CAD build for the part. Positions are in the model's coordinates, mm. A direction names the side the tool comes from. Round coordinates to 2 decimals unless told otherwise and drop trailing zeros. Loops run counter-clockwise (first coordinate to the right, second up) from the corner with the lowest first, then second, coordinate; pieces in that order, holes last.
from build123d import *

# Parameters (mm, degrees)
CROQUIS1_R              = 4.5
SALIENTE_EXTRUIR1_DEPTH = 12.5
SALIENTE_EXTRUIR2_START = 5
SALIENTE_EXTRUIR2_DEPTH = 5
CROQUIS4_R              = 2.5
SALIENTE_EXTRUIR3_DEPTH = 20
CORTAR_EXTRUIR1_DEPTH   = 3
SALIENTE_EXTRUIR4_START = -5
SALIENTE_EXTRUIR4_DEPTH = 5
CROQUIS7_W              = 256.925453937
CROQUIS7_H              = 4
CORTAR_EXTRUIR2_DEPTH   = 10
SALIENTE_EXTRUIR6_DEPTH = 5
CROQUIS9_W              = 256.997943919
CROQUIS9_H              = 4
CORTAR_EXTRUIR3_DEPTH   = 10
CROQUIS10_R             = 2.5
SALIENTE_EXTRUIR7_DEPTH = 25
SALIENTE_EXTRUIR9_DEPTH = 50
MATRIZL1_COUNT          = 2
MATRIZL1_PITCH          = 100
MATRIZL1_COPY_1_DEPTH   = 50


with BuildPart() as part:
    # Croquis1 → Saliente-Extruir1 (new, symmetric)
    with BuildSketch(Plane.XY):
        Circle(CROQUIS1_R)
    extrude(amount=SALIENTE_EXTRUIR1_DEPTH, both=True)

    # Croquis2 → Saliente-Extruir2 (add)
    with BuildSketch(Plane.XY.offset(12.5).offset(SALIENTE_EXTRUIR2_START)):
        with BuildLine():
            Line((0, 4.5), (120, 4.5))
            ThreePointArc((120, 4.5), (124.5, 0), (120, -4.5))
            Line((120, -4.5), (0, -4.5))
            ThreePointArc((0, -4.5), (-4.5, 0), (0, 4.5))
        make_face()
    saliente_extruir2 = extrude(amount=-SALIENTE_EXTRUIR2_DEPTH)

    # Simetría1: Saliente-Extruir2 across plane
    add(saliente_extruir2.mirror(Plane.XY))

    # Croquis4 → Saliente-Extruir3 (add, symmetric)
    with BuildSketch(Plane.XY):
        with Locations(Location((120, 0, 0), (0, 0, 180))):
            Circle(CROQUIS4_R)
    extrude(amount=SALIENTE_EXTRUIR3_DEPTH, both=True)

    # Croquis5 → Cortar-Extruir1 (cut)
    with BuildSketch(Plane.XY.offset(17.5)):
        with BuildLine():
            Line((0, 2), (90, 2))
            ThreePointArc((90, 2), (92, 0), (90, -2))
            Line((90, -2), (0, -2))
            ThreePointArc((0, -2), (-2, 0), (0, 2))
        make_face()
    cortar_extruir1 = extrude(amount=-CORTAR_EXTRUIR1_DEPTH, mode=Mode.SUBTRACT)

    # Simetría2: Cortar-Extruir1 across plane
    add(cortar_extruir1.mirror(Plane.XY), mode=Mode.SUBTRACT)

    # Croquis6 → Saliente-Extruir4 (add)
    with BuildSketch(Plane(origin=(0, 0, -17.5), x_dir=(-1, 0, 0), z_dir=(0, 0, -1)).offset(SALIENTE_EXTRUIR4_START)):
        with BuildLine():
            Line((0, 4.5), (210, 4.5))
            Line((210, 4.5), (210, -4.5))
            Line((210, -4.5), (0, -4.5))
            ThreePointArc((0, -4.5), (4.5, 0), (0, 4.5))
        make_face()
    extrude(amount=SALIENTE_EXTRUIR4_DEPTH)

    # Croquis7 → Cortar-Extruir2 (cut)
    with BuildSketch(Plane(origin=(0, 0, -14.5), x_dir=(-1, 0, 0), z_dir=(0, 0, -1))):
        with Locations((128.462726969, 0)):
            Rectangle(CROQUIS7_W, CROQUIS7_H)
    extrude(amount=CORTAR_EXTRUIR2_DEPTH, mode=Mode.SUBTRACT)

    # Croquis8 → Saliente-Extruir6 (add)
    with BuildSketch(Plane.XY.offset(17.5)):
        with BuildLine():
            Line((0, 4.5), (-210, 4.5))
            Line((-210, 4.5), (-210, -4.5))
            Line((-210, -4.5), (0, -4.5))
            ThreePointArc((0, -4.5), (-4.5, 0), (0, 4.5))
        make_face()
    extrude(amount=-SALIENTE_EXTRUIR6_DEPTH)

    # Croquis9 → Cortar-Extruir3 (cut)
    with BuildSketch(Plane.XY.offset(14.5)):
        with Locations((-128.49897196, 0)):
            Rectangle(CROQUIS9_W, CROQUIS9_H)
    extrude(amount=CORTAR_EXTRUIR3_DEPTH, mode=Mode.SUBTRACT)

    # Croquis10 → Saliente-Extruir7 (add)
    with BuildSketch(Plane.XY.offset(-12.5)):
        with Locations(Location((109.5, 0, 0), (0, 0, 180))):
            Circle(CROQUIS10_R)
        with Locations(Location((94.5, 0, 0), (0, 0, 180))):
            Circle(CROQUIS10_R)
        with Locations(Location((79.5, 0, 0), (0, 0, 180))):
            Circle(CROQUIS10_R)
        with Locations(Location((64.5, 0, 0), (0, 0, 180))):
            Circle(CROQUIS10_R)
        with Locations(Location((49.5, 0, 0), (0, 0, 180))):
            Circle(CROQUIS10_R)
        with Locations(Location((34.5, 0, 0), (0, 0, 180))):
            Circle(CROQUIS10_R)
        with Locations(Location((19.5, 0, 0), (0, 0, 180))):
            Circle(CROQUIS10_R)
    extrude(amount=SALIENTE_EXTRUIR7_DEPTH)

    # Croquis13 → Saliente-Extruir9 (add)
    with BuildSketch(Plane.ZY.offset(210)):
        with BuildLine():
            Line((17.5, 4.5), (12.5, 4.5))
            ThreePointArc((12.5, 4.5), (0, 9.538029883), (-12.5, 4.5))
            Line((-12.5, 4.5), (-17.5, 4.5))
            ThreePointArc((-17.5, 4.5), (0, 14.414141438), (17.5, 4.5))
        make_face()
    saliente_extruir9 = extrude(amount=-SALIENTE_EXTRUIR9_DEPTH)

    # Simetría3: Saliente-Extruir9 across plane
    add(saliente_extruir9.mirror(Plane.ZX))

    # MatrizL1: Saliente-Extruir9 ×2
    with Locations(*[(i * MATRIZL1_PITCH, 0, 0) for i in range(1, MATRIZL1_COUNT)]):
        add(saliente_extruir9)

    # MatrizL1 copy 1 sketch → MatrizL1 copy 1 (add)
    with BuildSketch(Plane.ZY.offset(110)):
        with BuildLine():
            Line((17.5, -4.5), (12.5, -4.5))
            ThreePointArc((12.5, -4.5), (0, -9.538029883), (-12.5, -4.5))
            Line((-12.5, -4.5), (-17.5, -4.5))
            ThreePointArc((-17.5, -4.5), (0, -14.414141438), (17.5, -4.5))
        make_face()
    extrude(amount=-MATRIZL1_COPY_1_DEPTH)


solid = part.part
Item 1: 3-axis set-ups, long thin cutter, end or side, ignore diameter. For faces 1 (the flat face through (-60, 11, 0)), 2 (the flat face through (-60, -10, 0)), 3 (the flat face through (-110, -10, 0)), 4 (the flat face through (-106, 0, -12.5)), 5 (the flat face through (63, 3, 12.5)): which of +Z, -Z, +X, -X, +Y, -Y reach the whole face in a straight line?
Verdict:
face 1: +Z, -Z, +X, +Y
face 2: +Z, -Z, +X, -Y
face 3: +Z, -Z, -Y
face 4: -X
face 5: none
Item 2: Cut at A-A (x = 26). List the corners of the cut face in (y, z), plus the area to 3 significant figures.
Verdict:
outline: (-4.5, -17.5) - (-2, -17.5) - (-2, -14.5) - (2, -14.5) - (2, -17.5) - (4.5, -17.5) - (4.5, -12.5) - (-4.5, -12.5) - close; (-4.5, 12.5) - (4.5, 12.5) - (4.5, 17.5) - (2, 17.5) - (2, 14.5) - (-2, 14.5) - (-2, 17.5) - (-4.5, 17.5) - close
area: 66.0 mm2
Item 3: Flat gauge pins, fed straight in: P1, Ø7, axis at x = -110.5, y = -2, coming from the +Z side; P2, Ø2.5, axis at x = 12, z = 14, coming from the +Y side; P3, Ø1, axis at y = 11, z = -2.5, coming from the +X side; P4, Ø1.5, axis at x = -53, y = -5.5, coming from the +Z side. Where does each tip first touch, or does it go through?
Verdict:
P1: stops at z = 17.5
P2: stops at y = 4.5
P3: stops at x = -60
P4: passes through
Item 4: Cut at B-B (z = -1.5). State how many separate pieces and enclosed holes the cut face has, plus the area to 3 significant figures.
Verdict:
separate pieces: 13
enclosed holes: 0
area: 1,200 mm2
Item 5: Wall check: L1, parallel to Y at x = -34.5, z = -15.5; L2, parallel to X at y = 10.5, z = -9; L3, parallel to Z at x = -79, y = -4. Give the ranges that are in metal, low to high.
Verdict:
L1: y = -4.5 to -2, 2 to 4.5
L2: x = -210 to -160, -110 to -60
L3: z = -17.5 to -12.5, 12.5 to 17.5
Item 6: Mould opens along Z. For faces 6 (the flat face through (-106, 0, 12.5)), 7 (the flat face through (-210, 9.4, 4.1)), 8 (the cylindrical face through (-85.35, -14.412, -0.294)) say: released by +Z, released by -Z, zero draft, split by the parting line, or undercut.
Verdict:
face 6: undercut
face 7: zero draft
face 8: split by the parting line
